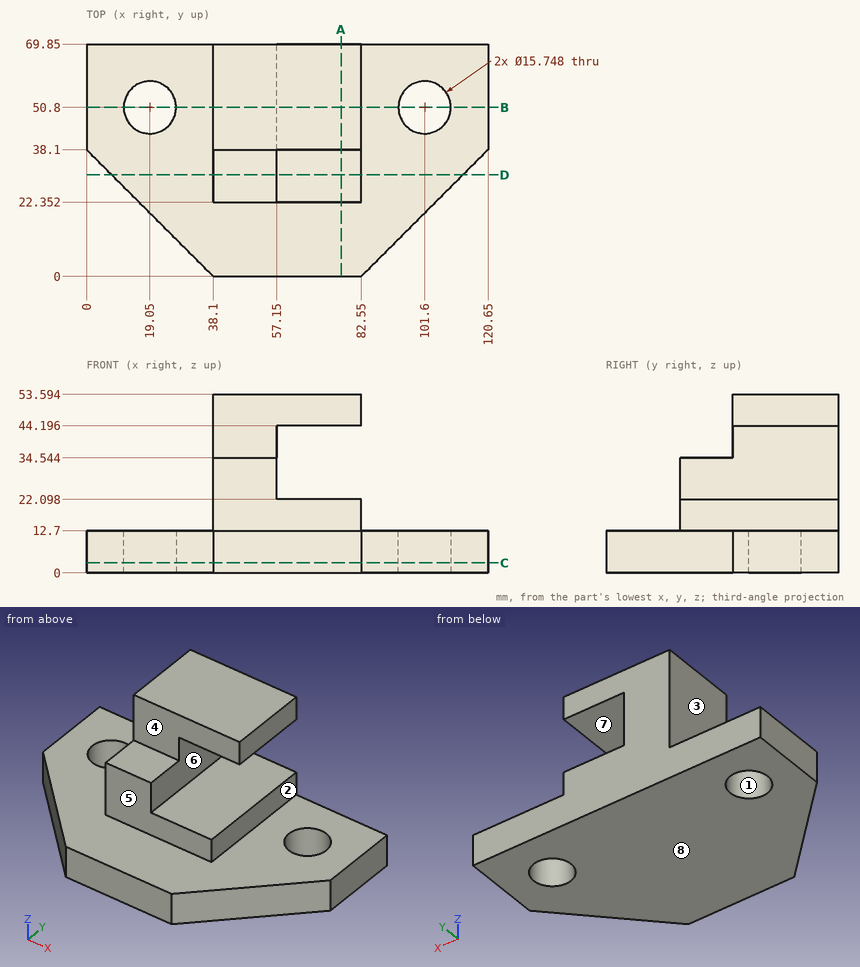
The figure shows three views and two pictorial views of one solid part (mm, origin at its lowest corner). Answer the questions. A direction names the side the tool comes from. Round coordinates to 2 decimals unless told otherwise and drop trailing zeros. Write each loop counter-clockwise with the first axis right and the second up, starting at its lowest first coordinate (ties: lowest second). Pieces come first, ordered by that corner, then holes. Notation, with made-up numbers: (-33, 88) - (0, 88) arc R22 cw to (0, 108) - close; hole circle Ø6 at (12, 87.5). An arc over 180 degrees is marked (long way). Answer in a Markdown table with one row per item. Add a question column.
1. A cutting plane is placed at C-C, the plane z = 3. Determine the outline of the cut face in (x, y), and give its area (3 significant figures).
2. A cutting plane is placed at D-D, the plane y = 30.5. Determine the outline of the cut face in (x, z), and give its area (3 significant figures).
3. Given pin 1 (3 mm diameter, centred on x = 37, y = 20, fed in from +Z); pin 2 (7.5 mm diameter, centred on y = 58.5, z = 48.5, fed in from +X); pin 3 (5.5 mm diameter, centred on x = 65.5, z = 41, fed in from -Y); pin 4 (11 mm diameter, centred on x = 60.5, z = 24.5, fed in from -Y), each flat-ended and moving along its own axis, determine where each tip first touches the part or whether it passes through.
4. For the marked faces 1, 2, 3 and 4, determine the directions among +Z, -Z, +X, -X, +Y, -Y from which every point of the face is accessible in a straight line to the end or side of a thin tool.
5. A cutting plane is placed at B-B, the plane y = 50.8. Determine the outline of the cut face in (x, z).
6. A cutting plane is placed at A-A, the plane x = 76.5. Determine the outline of the cut face in (y, z), and give its area (3 significant figures).
7. The mould has two halves that part along Z. Classify the marked faces 5, 6, 7 and 8: +Z half, -Z half, draft (parallel to the pull), parting line (faces both ways), or undercut.
8. Find the intervals of material crossed by line 1 along Z through (x, y) = (80, 56.5); line 2 along X through (y, z) = (53.5, 12.5); line 3 along X through (y, z) = (50, 4), in increasing order. Write a range as from..to.
Worked out:
| question | item | result |
|---|---|---|
| 1 | outline | (0, 38.1) - (38.1, 0) - (82.55, 0) - (120.65, 38.1) - (120.65, 69.85) - (0, 69.85) - close; hole circle Ø15.75 at (19.05, 50.8); hole circle Ø15.75 at (101.6, 50.8) |
| 1 | area | 6,590 mm^2 |
| 2 | outline | (7.6, 0) - (113.05, 0) - (113.05, 12.7) - (82.55, 12.7) - (82.55, 22.1) - (57.15, 22.1) - (57.15, 34.54) - (38.1, 34.54) - (38.1, 12.7) - (7.6, 12.7) - close |
| 2 | area | 1,990 mm^2 |
| 3 | pin 1 | z = 12.7 |
| 3 | pin 2 | x = 82.55 |
| 3 | pin 3 | through |
| 3 | pin 4 | y = 22.35 |
| 4 | face 1 | +Z, -Z |
| 4 | face 2 | +Z, +X, +Y, -Y |
| 4 | face 3 | +Z, -X, +Y, -Y |
| 4 | face 4 | +Z, +X, -X, -Y |
| 5 | outline | (0, 0) - (11.18, 0) - (11.18, 12.7) - (0, 12.7) - close; (26.92, 0) - (93.73, 0) - (93.73, 12.7) - (82.55, 12.7) - (82.55, 22.1) - (57.15, 22.1) - (57.15, 44.2) - (82.55, 44.2) - (82.55, 53.59) - (38.1, 53.59) - (38.1, 12.7) - (26.92, 12.7) - close; (109.47, 0) - (120.65, 0) - (120.65, 12.7) - (109.47, 12.7) - close |
| 6 | outline | (0, 0) - (69.85, 0) - (69.85, 22.1) - (22.35, 22.1) - (22.35, 12.7) - (0, 12.7) - close; (38.1, 44.2) - (69.85, 44.2) - (69.85, 53.59) - (38.1, 53.59) - close |
| 6 | area | 1,630 mm^2 |
| 7 | face 5 | draft |
| 7 | face 6 | undercut |
| 7 | face 7 | undercut |
| 7 | face 8 | -Z half |
| 8 | line 1 | 0..22.1, 44.2..53.59 |
| 8 | line 2 | 0..11.65, 26.45..94.2, 109..120.65 |
| 8 | line 3 | 0..11.22, 26.88..93.77, 109.43..120.65 |
